Geometry check sheet. Reference: the model listing, model coordinates, mm. A direction names the side the tool comes from. Give positions to 0.01 mm unless a question says otherwise; leave off trailing zeros. Loops run counter-clockwise (first coordinate to the right, second up) from the corner with the lowest first, then second, coordinate; pieces in that order, holes last. Notation, with made-up numbers: (-5, 83.25) -> (45, 83.25) arc R21 ccw to (45, 117.25) -> close; hole circle Ø2 at (52.5, 66.25). An arc over 180 degrees is marked (long way). One line per question, with ' | ' between items.
from build123d import *

# Parameters (mm, degrees)
F1_DEPTH = 3.175


# Not quite as in the source:
# - a length typed as a fraction of an inch, garbled in the dataset ("3 / 203.2 mm" for 3/8 in), is restored


with BuildPart() as f1:
    # F0 (on Top) → F1 (new body)
    with BuildSketch(Plane.XY):
        with BuildLine():
            Line((50.8, 0), (25.4, 66.475))
            Line((25.4, 66.475), (-25.4, 66.475))
            Line((-25.4, 66.475), (-50.8, 0))
            Line((-50.8, 0), (-50.8, -47.825))
            Line((-50.8, -47.825), (-34.925, -47.825))
            Line((-34.925, -47.825), (-34.925, -98.625))
            Line((-34.925, -98.625), (-25.4, -98.625))
            ThreePointArc((-25.4, -98.625), (0, -73.225), (25.4, -98.625))
            Line((25.4, -98.625), (34.925, -98.625))
            Line((34.925, -98.625), (34.925, -47.825))
            Line((34.925, -47.825), (50.8, -47.825))
            Line((50.8, -47.825), (50.8, 0))
        make_face()
    extrude(amount=-F1_DEPTH)


solid = f1.part
Item 1: Sectioned sample at A-A (y = -75.5). Record the cut outline in (x, z) (3 decimals).
Result:
outline: (-34.925, -3.175) -> (-10.507, -3.175) -> (-10.507, 0) -> (-34.925, 0) -> close; (10.507, -3.175) -> (34.925, -3.175) -> (34.925, 0) -> (10.507, 0) -> close
Item 2: Set-up check for faces 1 (the face through (34.925, -74, -2)), 2 (the face through (-50.8, -24, -2)), 3 (the face through (-43, -47.825, -2)): record each of +Z, -Z, +X, -X, +Y, -Y from which the full face is reachable in a straight line by a thin tool's end or side.
Result:
face 1: +Z, -Z, +X, -Y | face 2: +Z, -Z, -X, +Y, -Y | face 3: +Z, -Z, -X, -Y
Item 3: Sectioned sample at D-D (y = 49). Record the cut outline in (x, z) (3 decimals), plus the area to 3 significant figures.
Result:
outline: (-32.077, -3.175) -> (32.077, -3.175) -> (32.077, 0) -> (-32.077, 0) -> close | area: 204 mm2
Item 4: Release check for a two-part mould opening along X. For faces 4 (the face through (38.28, 32.77, -1.57)), 5 (the face through (-34.925, -73, -2)), 6 (the face through (-0.56, -73.23, -1.57)) record: pulls with the +X half, pulls with the -X half, needs draft (parallel to the pull), parting line crosses it, or undercut.
Result:
face 4: pulls with the +X half | face 5: pulls with the -X half | face 6: undercut
Item 5: Depth check by flat-ended pin: pin 1 Ø1.6 at (x, z) = (-40, -1) entering from -Y (3 decimals); pin 2 Ø1 at (y, z) = (-63.5, -2) entering from +X (3 decimals). Enter the tip coordinate at first touch or a pass-through.
Result:
pin 1: y = -47.825 | pin 2: x = 34.925
Item 6: Sectioned sample at B-B (z = -2.2). Record the cut outline in (x, y) (3 decimals), plus the area to 3 significant figures.
Result:
outline: (-50.8, -47.825) -> (-34.925, -47.825) -> (-34.925, -98.625) -> (-25.4, -98.625) arc R25.4 cw to (25.4, -98.625) -> (34.925, -98.625) -> (34.925, -47.825) -> (50.8, -47.825) -> (50.8, 0) -> (25.4, 66.475) -> (-25.4, 66.475) -> (-50.8, 0) -> close | area: 12,500 mm2
Item 7: Scan lines: probe 1 along X at (y, z) = (-68.5, -2.35) (3 decimals); probe 2 along X at (y, z) = (-90, -0.15) (3 decimals); probe 3 along Y at (x, z) = (11.5, -2.35) (3 decimals). Record each from-to range of solid material in increasing order.
Result:
probe 1: -34.925 to 34.925 | probe 2: -34.925 to -23.891, 23.891 to 34.925 | probe 3: -75.977 to 66.475
Item 8: Sectioned sample at C-C (x = 0). Record the cut outline in (y, z) (3 decimals), plus the area to 3 significant figures.
Result:
outline: (-73.225, -3.175) -> (66.475, -3.175) -> (66.475, 0) -> (-73.225, 0) -> close | area: 444 mm2
